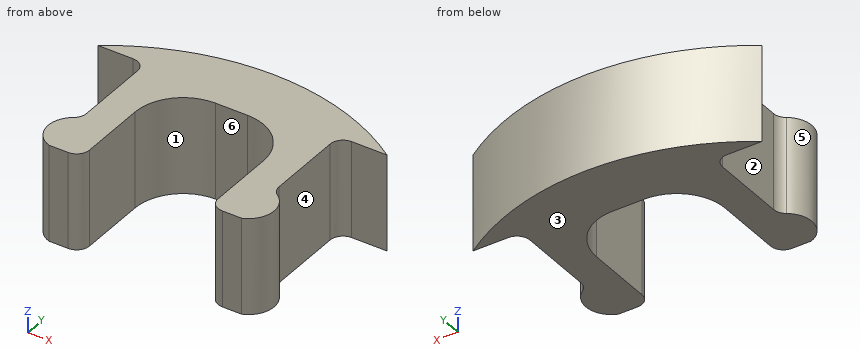
from build123d import *

# Parameters (mm, degrees)
DODANIE_WYCI_GNI_CIE1_DEPTH = 3
ZAOKR_GLENIE2_R             = 0.4
ZAOKR_GLENIE3_R             = 1.5


with BuildPart() as part:
    # Szkic1 → Dodanie-wyciągnięcie1 (new body)
    with BuildSketch(Plane.XY):
        with BuildLine():
            Line((0, 3), (-1.5, 3))
            ThreePointArc((-1.5, 3), (3, 4.425195836), (7.5, 3))
            Line((7.5, 3), (6, 3))
            Line((6, 3), (6, -0.005902175))
            ThreePointArc((6, -0.005902175), (6.513786929, -0.752951087), (6, -1.5))
            Line((6, -1.5), (5, -1.5))
            Line((5, -1.5), (5, 2.5))
            Line((5, 2.5), (1, 2.5))
            Line((1, 2.5), (1, -1.5))
            Line((1, -1.5), (0, -1.5))
            ThreePointArc((0, -1.5), (-0.521611782, -0.75), (0, 0))
            Line((0, 0), (0, 3))
        make_face()
    extrude(amount=DODANIE_WYCI_GNI_CIE1_DEPTH)

    # Zaokrąglenie2
    zaokr_glenie2_edges = [part.edges().sort_by_distance(p)[0] for p in [
        (0, 0, 1.5),
        (0, 3, 1.5),
        (6, 3, 1.5),
        (6, -0.005902175, 1.5),
        (5, -1.5, 1.5),
        (1, -1.5, 1.5),
    ]]
    fillet(zaokr_glenie2_edges, radius=ZAOKR_GLENIE2_R)

    # Zaokrąglenie3
    zaokr_glenie3_edges = [part.edges().sort_by_distance(p)[0] for p in [
        (5, 2.5, 1.5),
        (1, 2.5, 1.5),
    ]]
    fillet(zaokr_glenie3_edges, radius=ZAOKR_GLENIE3_R)


solid = part.part
Here's how the part is built. I have some questions about the finished solid (model axes, mm). Face numbers are marked on the shaded views. A direction names the side the tool comes from. Round coordinates to 2 decimals unless told otherwise and drop trailing zeros. Write each loop counter-clockwise with the first axis right and the second up, starting at its lowest first coordinate (ties: lowest second). Pieces come first, ordered by that corner, then holes.
1. Suppose I cut it at B-B (z = 2.65). List the corners of the cut face in (x, y) for me.
2. Will these pins go through, and if not, where does the flat tip stop? pin 1 Ø1.1 at (x, z) = (3, 1) entering from -Y; pin 2 Ø0.5 at (x, z) = (7, 1.5) entering from -Y; pin 3 Ø1.7 at (y, z) = (0.5, 2) entering from -X.
3. If we mould it in two halves opening along Y, with no side actions, what happens to the marked faces 1, 2 and 3? For each: released by +Y, released by -Y, zero draft, split by the parting line, or undercut.
4. Suppose I cut it at A-A (y = 0.9). List the corners of the cut face in (x, z) for me.
5. Suppose I cut it at C-C (y = 2.2). List the corners of the cut face in (x, z) for me.
6. I need wall thicknesses on L1, parallel to X at y = -0.7, z = 1.7; L2, parallel to X at y = 0.3, z = 1; L3, parallel to Y at x = 2.25, z = 0.85. Which ranges of each line are inside material? Lowest first, please.
7. Suppose I cut it at D-D (x = 4.75). List the corners of the cut face in (y, z) for me.
8. For the marked faces 4, 5 and 6, which set-ups out of +Z, -Z, +X, -X, +Y, -Y let a thin tool reach every point of the face, with its end or its side?
Answer sheet:
1. outline: (-1.5, 3) - (-0.4, 3) arc R0.4 cw to (0, 2.6) - (0, 0.24) arc R0.4 cw to (-0.17, -0.09) arc R0.8 ccw to (0, -1.5) - (0.6, -1.5) arc R0.4 ccw to (1, -1.1) - (1, 1) arc R1.5 cw to (2.5, 2.5) - (3.5, 2.5) arc R1.5 cw to (5, 1) - (5, -1.1) arc R0.4 ccw to (5.4, -1.5) - (6, -1.5) arc R0.8 ccw to (6.17, -0.1) arc R0.4 cw to (6, 0.23) - (6, 2.6) arc R0.4 cw to (6.4, 3) - (7.5, 3) arc R7.82 ccw to start
2. pin 1: stops at y = 2.5
2. pin 2: stops at y = 3
2. pin 3: stops at x = -0.41
3. face 1: released by -Y
3. face 2: undercut
3. face 3: zero draft
4. outline: (0, 0) - (1, 0) - (1, 3) - (0, 3) - close; (5, 0) - (6, 0) - (6, 3) - (5, 3) - close
5. outline: (0, 0) - (1.6, 0) - (1.6, 3) - (0, 3) - close; (4.4, 0) - (6, 0) - (6, 3) - (4.4, 3) - close
6. L1: x = -0.52 to 1, 5 to 6.51
6. L2: x = 0 to 1, 5 to 6
6. L3: y = 2.48 to 4.39
7. outline: (1.83, 0) - (4.23, 0) - (4.23, 3) - (1.83, 3) - close
8. face 4: +Z, -Z, +X
8. face 5: +Z, -Z, -X
8. face 6: +Z, -Z, -Y
